Read the model definition and answer for the solid it produces. Units are mm, in the model's axes. A direction names the side the tool comes from. Coordinates: 2 decimals unless noted, no trailing zeros. Order: outer loops, then holes, each group sorted by start corner. A loop starts at its lowest first (then second) coordinate and runs counter-clockwise, first axis right, second up. Notation, with made-up numbers: (60, -21) - (101, -21) arc R23 cw to (101, -5) - close; hole circle Ø2 at (-21.5, -14.75). An arc over 180 degrees is marked (long way). Use one line per item in the form item = value.
```python
from build123d import *

# Parameters (mm, degrees)
SKETCH1_R           = 6.5
SKETCH1_R_2         = 1.5
BOSS_EXTRUDE1_DEPTH = 8.636
FILLET1_R           = 12.7
FILLET2_R           = 1.27


with BuildPart() as part:
    # Sketch1 → Boss-Extrude1 (new body)
    with BuildSketch(Plane.XY):
        Polygon((0, 0), (88.9, 0), (88.9, 9.525), (75.6412, 9.525), (75.6412, 50.8), (13.25, 50.8), (13.25, 9.525), (0, 9.525), align=None)
        with Locations((44.45, 32.4)):
            Circle(SKETCH1_R, mode=Mode.SUBTRACT)
        with Locations((28.95, 25.4)):
            Circle(SKETCH1_R_2, mode=Mode.SUBTRACT)
        with Locations((59.95, 25.4)):
            Circle(SKETCH1_R_2, mode=Mode.SUBTRACT)
        with Locations((52.2, 11.976606241)):
            Circle(SKETCH1_R_2, mode=Mode.SUBTRACT)
        with Locations((36.7, 11.976606241)):
            Circle(SKETCH1_R_2, mode=Mode.SUBTRACT)
        with Locations((36.7, 38.823393759)):
            Circle(SKETCH1_R_2, mode=Mode.SUBTRACT)
        with Locations((52.2, 38.823393759)):
            Circle(SKETCH1_R_2, mode=Mode.SUBTRACT)
    extrude(amount=BOSS_EXTRUDE1_DEPTH)

    # Fillet1
    fillet1_edges = [part.edges().sort_by_distance(p)[0] for p in [
        (13.25, 50.8, 4.318),
        (75.6412, 50.8, 4.318),
    ]]
    fillet(fillet1_edges, radius=FILLET1_R)

    # Fillet2
    fillet2_edges = [part.edges().sort_by_distance(p)[0] for p in [
        (0, 9.525, 4.318),
        (13.25, 9.525, 4.318),
        (75.6412, 9.525, 4.318),
        (88.9, 9.525, 4.318),
    ]]
    fillet(fillet2_edges, radius=FILLET2_R)


solid = part.part
```
(1) Section A-A, the plane x = 59.95 is taken. Write down the section's boundary in (y, z), then the cut area to 3 significant figures.
Answer list:
outline = (0, 0) - (23.9, 0) - (23.9, 8.64) - (0, 8.64) - close; (26.9, 0) - (50.8, 0) - (50.8, 8.64) - (26.9, 8.64) - close
area = 413 mm2
(2) The mould has two halves that part along X. Classify faces 4 (the cylindrical face through (51.87, 37.36, 4.26)), 5 (the flat face through (44, 0, 4)), 6 (the flat face through (0, 4, 4)): +X half, -X half, draft (parallel to the pull), parting line (faces both ways), or undercut.
Answer list:
face_4 = undercut
face_5 = draft
face_6 = -X half
(3) Section B-B, the plane x = 36.7 is taken. Write down the section's boundary in (y, z).
Answer list:
outline = (0, 0) - (10.48, 0) - (10.48, 8.64) - (0, 8.64) - close; (13.48, 0) - (37.32, 0) - (37.32, 8.64) - (13.48, 8.64) - close; (40.32, 0) - (50.8, 0) - (50.8, 8.64) - (40.32, 8.64) - close
(4) Section D-D, the plane z = 1 is taken. Write down the section's boundary in (x, y) (3 decimals), then the cut area to 3 significant figures.
Answer list:
outline = (0, 0) - (88.9, 0) - (88.9, 8.255) arc R1.27 ccw to (87.63, 9.525) - (76.911, 9.525) arc R1.27 cw to (75.641, 10.795) - (75.641, 38.1) arc R12.7 ccw to (62.941, 50.8) - (25.95, 50.8) arc R12.7 ccw to (13.25, 38.1) - (13.25, 10.795) arc R1.27 cw to (11.98, 9.525) - (1.27, 9.525) arc R1.27 ccw to (0, 8.255) - close; hole circle Ø3 at (28.95, 25.4); hole circle Ø3 at (36.7, 11.977); hole circle Ø3 at (36.7, 38.823); hole circle Ø13 at (44.45, 32.4); hole circle Ø3 at (52.2, 11.977); hole circle Ø3 at (52.2, 38.823); hole circle Ø3 at (59.95, 25.4)
area = 3,180 mm2
(5) Section C-C, the plane y = 30.5 is taken. Write down the section's boundary in (x, z).
Answer list:
outline = (13.25, 0) - (38.23, 0) - (38.23, 8.64) - (13.25, 8.64) - close; (50.67, 0) - (75.64, 0) - (75.64, 8.64) - (50.67, 8.64) - close
(6) Straight lines are drawn through the part: L1, parallel to Y at x = 52.2, z = 5.75; L2, parallel to X at y = 12, z = 3.25; L3, parallel to Y at x = 28.95, z = 3.5. For each, find the intervals that lie inside material, in ascending order.
Answer list:
L1 = 0 to 10.48, 13.48 to 37.32, 40.32 to 50.8
L2 = 13.25 to 35.2, 38.2 to 50.7, 53.7 to 75.64
L3 = 0 to 23.9, 26.9 to 50.8
(7) Given pin 1 Ø3.5 at (x, y) = (36.7, 11.98) entering from +Z; pin 2 Ø11.5 at (x, y) = (44.45, 32.4) entering from -Z; pin 3 Ø5 at (y, z) = (32.5, 5) entering from -X; pin 4 Ø1.5 at (y, z) = (29.5, 1.5) entering from +X, each flat-ended and moving along its own axis, determine where each tip first touches the part or whether it passes through.
Answer list:
pin_1 = 8.64
pin_2 = through
pin_3 = 13.25
pin_4 = 75.64
(8) Which of the six approach directions +Z, -Z, +X, -X, +Y, -Y give full straight-line access (tool end or side, diameter ignored) to faces 1 (the flat face through (82, 9.525, 4)), 2 (the flat face through (45, 50.8, 4)), 3 (the flat face through (13.25, 25, 4))?
Answer list:
face_1 = +Z, -Z, +X, +Y
face_2 = +Z, -Z, +X, -X, +Y
face_3 = +Z, -Z, -X, +Y
